Geometry check sheet. Reference: the model listing, model coordinates, mm. A direction names the side the tool comes from. Coordinates: 2 decimals unless noted, no trailing zeros. Write each loop counter-clockwise with the first axis right and the second up, starting at its lowest first coordinate (ties: lowest second). Pieces come first, ordered by that corner, then holes. Notation, with made-up numbers: (72, 64) -> (107, 64) arc R18 ccw to (107, 73) -> close; hole circle Ø5 at (-25.5, 30). An arc over 180 degrees is marked (long way). Use a Markdown table: item, result.
```python
from build123d import *

# Parameters (mm, degrees)
BOSS_EXTRUDE1_DEPTH = 20
SKETCH2_R           = 5
CUT_EXTRUDE1_DEPTH  = 16
FILLET1_R           = 400


with BuildPart() as part:
    # Sketch1 → Boss-Extrude1 (new body)
    with BuildSketch(Plane(origin=(0, 0, 0), x_dir=(1, 0, 0), z_dir=(0, 1, 0))):
        with BuildLine():
            ThreePointArc((12.5, 156.5), (0, 169), (-12.5, 156.5))
            Line((-12.5, 156.5), (-5, 156.5))
            ThreePointArc((-5, 156.5), (0, 161.5), (5, 156.5))
            Line((5, 156.5), (12.5, 156.5))
        make_face()
        with BuildLine():
            Line((-5, 156.5), (-12.5, 156.5))
            ThreePointArc((-12.5, 156.5), (0, 144), (12.5, 156.5))
            Line((12.5, 156.5), (5, 156.5))
            ThreePointArc((5, 156.5), (0, 151.5), (-5, 156.5))
        make_face()
        with BuildLine():
            Line((-12.5, 156.5), (-12.5, 96.44212153))
            Line((-12.5, 96.44212153), (12.5, 96.44212153))
            Line((12.5, 96.44212153), (12.5, 156.5))
            ThreePointArc((12.5, 156.5), (0, 144), (-12.5, 156.5))
        make_face()
        Polygon((-12.5, 96.44212153), (-25, 7.5), (-2.3e-08, 7.5), (25, 7.5), (12.5, 96.44212153), align=None)
        with BuildLine():
            Line((-2.3e-08, 7.5), (-25, 7.5))
            Line((-25, 7.5), (-45, 7.5))
            Line((-45, 7.5), (-45, -7.5))
            Line((-45, -7.5), (-15, -7.5))
            ThreePointArc((-15, -7.5), (-10.606601726, 3.10660171), (-2.3e-08, 7.5))
        make_face()
        with BuildLine():
            Line((25, 7.5), (-2.3e-08, 7.5))
            ThreePointArc((-2.3e-08, 7.5), (10.60660171, 3.106601726), (15, -7.5))
            Line((15, -7.5), (45, -7.5))
            Line((45, -7.5), (45, 7.5))
            Line((45, 7.5), (25, 7.5))
        make_face()
    extrude(amount=BOSS_EXTRUDE1_DEPTH)

    # Sketch2 → Cut-Extrude1 (cut, through all)
    with BuildSketch(Plane(origin=(0, 0, -7.5), x_dir=(-1, 0, 0), z_dir=(0, 0, -1))):
        with Locations((35, 10)):
            Circle(SKETCH2_R)
        with Locations((-35, 10)):
            Circle(SKETCH2_R)
    extrude(amount=-CUT_EXTRUDE1_DEPTH, mode=Mode.SUBTRACT)

    # Fillet1
    fillet1_edges = [part.edges().sort_by_distance(p)[0] for p in [
        (12.5, 10, -96.44212153),
        (-12.5, 10, -96.44212153),
    ]]
    fillet(fillet1_edges, radius=FILLET1_R)


solid = part.part
```
Item 1: Thickness scan on L1, parallel to Y at x = -35, z = 1; L2, parallel to Z at x = -0.5, y = 4; L3, parallel to Z at x = 30, y = 1.5. Record the ranges inside material, lowest first. Write a range as [from, to].
Answer block:
| item | result |
|---|---|
| L1 | y = [0, 5], [15, 20] |
| L2 | z = [-168.99, -161.47], [-151.53, -7.49] |
| L3 | z = [-7.5, 7.5] |
Item 2: Depth check by flat-ended pin: P1, Ø8, axis at y = 3, z = -58, coming from the +X side; P2, Ø10, axis at x = -33.5, y = 6.5, coming from the -Z side; P3, Ø1, axis at y = 2.5, z = -10.5, coming from the -X side; P4, Ø9, axis at x = -35, y = 10, coming from the -Z side. Enter the tip coordinate at first touch or a pass-through.
Answer block:
| item | result |
|---|---|
| P1 | stops at x = 18.46 |
| P2 | stops at z = -7.5 |
| P3 | stops at x = -24.65 |
| P4 | passes through |
Item 3: Tool access check on faces 1 (the flat face through (12.5, 10, -140)), 2 (the flat face through (-12.5, 10, -141)), 3 (the flat face through (-1, 0, -62)). Record the directions out of +Z, -Z, +X, -X, +Y, -Y that give a thin tool (end or side, any length) a straight path to the whole face; none if there is none.
Answer block:
| item | result |
|---|---|
| face 1 | -Z, +X, +Y, -Y |
| face 2 | -Z, -X, +Y, -Y |
| face 3 | +Z, -Z, +X, -X, -Y |
Item 4: Section check D-D on x = 18. Record the boundary of the cut face in (y, z).
Answer block:
| item | result |
|---|---|
| outline | (0, -57.31) -> (20, -57.31) -> (20, 7.5) -> (0, 7.5) -> close |
Item 5: Section check C-C on z = -148. Record the boundary of the cut face in (x, y), then the cut area to 3 significant figures.
Answer block:
| item | result |
|---|---|
| outline | (-12.5, 0) -> (12.5, 0) -> (12.5, 20) -> (-12.5, 20) -> close |
| area | 500 mm^2 |
Item 6: Section check B-B on x = -35. Record the boundary of the cut face in (y, z).
Answer block:
| item | result |
|---|---|
| outline | (0, -7.5) -> (5, -7.5) -> (5, 7.5) -> (0, 7.5) -> close; (15, -7.5) -> (20, -7.5) -> (20, 7.5) -> (15, 7.5) -> close |
Item 7: Section check A-A on y = 10. Record the boundary of the cut face in (x, z).
Answer block:
| item | result |
|---|---|
| outline | (-45, -7.5) -> (-40, -7.5) -> (-40, 7.5) -> (-45, 7.5) -> close; (-30, -7.5) -> (-25, -7.5) -> (-16.39, -68.74) arc R400 cw to (-12.5, -124.41) -> (-12.5, -156.5) arc R12.5 ccw to (12.5, -156.5) -> (12.5, -124.41) arc R400 cw to (16.39, -68.74) -> (25, -7.5) -> (30, -7.5) -> (30, 7.5) -> (15, 7.5) arc R15 cw to (-15, 7.5) -> (-30, 7.5) -> close; (40, -7.5) -> (45, -7.5) -> (45, 7.5) -> (40, 7.5) -> close; hole circle Ø10 at (0, -156.5) |
Item 8: Mould release check, pull along X, two halves, no side actions. Record for faces 4 (the flat face through (-45, 10, 0)), 5 (the cylindrical face through (-30, 10, 0)), 6 (the flat face through (29.8, 9.9, 7.5)): +X half, -X half, draft (parallel to the pull), parting line (faces both ways), or undercut.
Answer block:
| item | result |
|---|---|
| face 4 | -X half |
| face 5 | undercut |
| face 6 | draft |
